Source: CAD feature listing. Evaluate the final solid. Frame: model axes, mm. A direction names the side the tool comes from. Round coordinates to 2 decimals unless told otherwise and drop trailing zeros. Loops run counter-clockwise (first coordinate to the right, second up) from the corner with the lowest first, then second, coordinate; pieces in that order, holes last. Notation, with made-up numbers: (-36, 1.25) -> (-20, 1.25) arc R31 ccw to (-20, 29.25) -> close; hole circle Ø7 at (69.5, -26.5). An arc over 180 degrees is marked (long way). Write item = value, one per line.
from build123d import *

# Parameters (mm, degrees)
PAD065_DEPTH      = 1.5
PAD065_DEPTH_BACK = 31
POCKET022_DEPTH   = 42.751
POCKET023_DEPTH   = 6
POCKET024_DEPTH   = 6.501


with BuildPart() as part:
    # Sketch105 → Pad065 (new body, two sides)
    with BuildSketch(Plane(origin=(0, 0, 0), x_dir=(0, -1, 0), z_dir=(-1, 0, 0))) as pad065_sk:
        Polygon((-58, 1.6), (-244, 1.6), (-244, 44.35), (-232.15, 44.35), (-232.15, 42.35), (-92, 42.35), (-92, 44.35), (-88, 44.35), (-88, 8.1), (-58, 8.1), align=None)
    extrude(amount=PAD065_DEPTH)
    extrude(pad065_sk.sketch, amount=-PAD065_DEPTH_BACK)

    # Sketch106 (on Face1 of Pad065) → Pocket022 (cut, through all)
    with BuildSketch(Plane.YX.offset(-1.6)):
        Polygon((48.3023801265, -11.1976198735), (92, 32.5), (92, 11), (232.15, 11), (232.15, 27), (240.15, 27), (258.8163982142, 8.3336017858), (258.8163982142, 61.252958), (48.3023801265, 61.252958), align=None)
    extrude(amount=-POCKET022_DEPTH, mode=Mode.SUBTRACT)

    # Sketch107 (on Face17 of Pocket022) → Pocket023 (cut)
    with BuildSketch(Plane(origin=(0, 0, 44.35), x_dir=(0, -1, 0), z_dir=(0, 0, 1))):
        Polygon((-249.5028966484, 34.5330350464), (-249.5028966484, 9.6471033517), (-224.6169649536, 34.5330350464), align=None)
    extrude(amount=-POCKET023_DEPTH, mode=Mode.SUBTRACT)

    # Sketch108 (on Face13 of Pocket023) → Pocket024 (cut, through all)
    with BuildSketch(Plane(origin=(0, 0, 8.1), x_dir=(0, -1, 0), z_dir=(0, 0, 1))):
        Polygon((-88, 16.9), (-88, 3.7), (-79, 3.7), (-70.6961965864, 7.6606626805), (-79.9355339059, 16.9), align=None)
    extrude(amount=-POCKET024_DEPTH, mode=Mode.SUBTRACT)


solid = part.part
1. Contact query for flat-ended pins moving along their axis: pin 1 Ø4 at (x, y) = (3, 83.5) entering from +Z; pin 2 Ø6 at (x, y) = (5.5, 138.5) entering from +Z; pin 3 Ø2 at (y, z) = (82, 4) entering from +X. Output: stop coordinate, or through.
Evaluation:
pin_1 = 8.1
pin_2 = 42.35
pin_3 = 23.5
2. Set-up query: faces 4 (the face through (27, 236, 20)), 5 (the face through (12.216, 75.251, 4.896)), 6 (the face through (20.99, 238.16, 41.39)). Return all of +Z, -Z, +X, -X, +Y, -Y with unobstructed straight access to the full face (end or side cutting, diameter ignored); none if empty.
Evaluation:
face_4 = +Z, -Z, +X, +Y
face_5 = +Z, -Z
face_6 = +Z, +X, +Y
3. Section query B-B (z = 6.5). Return the cut outline in (x, y).
Evaluation:
outline = (-1.5, 58) -> (31, 90.5) -> (31, 92) -> (11, 92) -> (11, 232.15) -> (27, 232.15) -> (27, 240.15) -> (23.15, 244) -> (-1.5, 244) -> close; hole (3.7, 79) -> (7.66, 70.7) -> (16.9, 79.94) -> (16.9, 88) -> (3.7, 88) -> close
4. Section query A-A (x = 18.5). Return the cut outline in (y, z).
Evaluation:
outline = (78, 1.6) -> (92, 1.6) -> (92, 44.35) -> (88, 44.35) -> (88, 8.1) -> (78, 8.1) -> close; (232.15, 1.6) -> (244, 1.6) -> (244, 38.35) -> (240.65, 38.35) -> (240.65, 44.35) -> (232.15, 44.35) -> close
5. Line query: probe 1 along Y at (x, z) = (21, 38); probe 2 along Y at (x, z) = (0.5, 9.5); probe 3 along Z at (x, y) = (2.5, 78.5). Output: solid intervals per line, ascending. Write a range as from..to.
Evaluation:
probe_1 = 88..92, 232.15..244
probe_2 = 88..244
probe_3 = 1.6..8.1
6. Mould query, pull axis X, two halves, no side actions, for faces 1 (the face through (19, 232.15, 23)), 2 (the face through (11, 161, 22)), 3 (the face through (16.9, 84, 5)). Classes: released by +X, released by -X, zero draft, split by the parting line, or undercut.
Evaluation:
face_1 = zero draft
face_2 = released by +X
face_3 = undercut
7. Section query D-D (y = 144). Return the cut outline in (x, z).
Evaluation:
outline = (-1.5, 1.6) -> (11, 1.6) -> (11, 42.35) -> (-1.5, 42.35) -> close
8. Section query C-C (z = 40). Return the cut outline in (x, y), then the cut area to 3 significant figures.
Evaluation:
outline = (-1.5, 88) -> (28.5, 88) -> (31, 90.5) -> (31, 92) -> (11, 92) -> (11, 232.15) -> (27, 232.15) -> (15.15, 244) -> (-1.5, 244) -> close
area = 2,150 mm²
